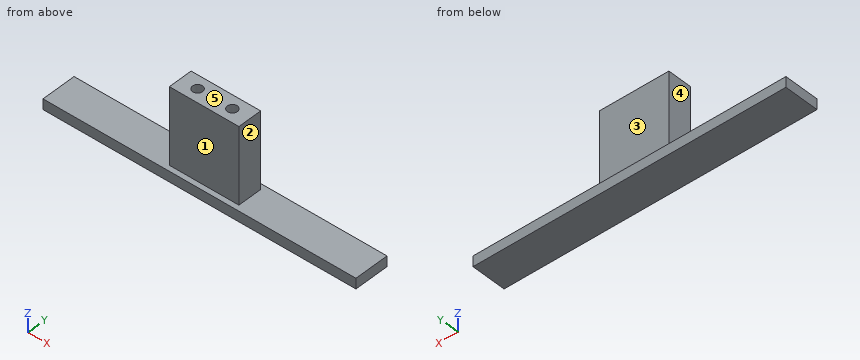
```python
from build123d import *

# Parameters (mm, degrees)
SKETCH_1_W          = 90
SKETCH_1_H          = 10
EXTRUDE_1_DEPTH     = 3
SKETCH_2_W          = 20
SKETCH_2_H          = 7
EXTRUDE_3_DEPTH     = 22
CUT_EXTRUDE_1_DEPTH = 9


with BuildPart() as part:
    # 草图1 → 凸台-拉伸1 (new body)
    with BuildSketch(Plane.XY):
        with Locations((45, 5)):
            Rectangle(SKETCH_1_W, SKETCH_1_H)
    extrude(amount=EXTRUDE_1_DEPTH)

    # 草图2 → 凸台-拉伸3 (add)
    with BuildSketch(Plane.XY.offset(3)):
        with Locations((45, 5)):
            Rectangle(SKETCH_2_W, SKETCH_2_H)
    extrude(amount=EXTRUDE_3_DEPTH)

    # 草图4 → 切除-拉伸1 (cut)
    with BuildSketch(Plane.XY.offset(25)):
        with BuildLine():
            ThreePointArc((48.55, 5), (50, 3.55), (51.45, 5))
            Line((51.45, 5), (50, 5))
            Line((50, 5), (48.55, 5))
        make_face()
        with BuildLine():
            Line((50, 5), (51.45, 5))
            ThreePointArc((51.45, 5), (50, 6.45), (48.55, 5))
            Line((48.55, 5), (50, 5))
        make_face()
        with BuildLine():
            ThreePointArc((48.55, 5), (50, 3.55), (51.45, 5))
            Line((51.45, 5), (50, 5))
            Line((50, 5), (48.55, 5))
        make_face()
        with BuildLine():
            Line((50, 5), (51.45, 5))
            ThreePointArc((51.45, 5), (50, 6.45), (48.55, 5))
            Line((48.55, 5), (50, 5))
        make_face()
        with BuildLine():
            ThreePointArc((38.55, 5), (40, 3.55), (41.45, 5))
            Line((41.45, 5), (40, 5))
            Line((40, 5), (38.55, 5))
        make_face()
        with BuildLine():
            Line((40, 5), (41.45, 5))
            ThreePointArc((41.45, 5), (40, 6.45), (38.55, 5))
            Line((38.55, 5), (40, 5))
        make_face()
        with BuildLine():
            ThreePointArc((38.55, 5), (40, 3.55), (41.45, 5))
            Line((41.45, 5), (40, 5))
            Line((40, 5), (38.55, 5))
        make_face()
        with BuildLine():
            Line((40, 5), (41.45, 5))
            ThreePointArc((41.45, 5), (40, 6.45), (38.55, 5))
            Line((38.55, 5), (40, 5))
        make_face()
    extrude(amount=-CUT_EXTRUDE_1_DEPTH, mode=Mode.SUBTRACT)


solid = part.part
```
CAD build for the part. Positions are in the model's coordinates, mm. Face numbers are marked on the shaded views. A direction names the side the tool comes from. Round coordinates to 2 decimals unless told otherwise and drop trailing zeros. Order: outer loops, then holes, each group sorted by start corner. A loop starts at its lowest first (then second) coordinate and runs counter-clockwise, first axis right, second up.
Item 1: Pin check, flat tips, straight feed: pin 1 (2 mm diameter, centred on y = 4.5, z = 11, fed in from -X); pin 2 (5 mm diameter, centred on x = 78.5, y = 7.5, fed in from +Z); pin 3 (0.9 mm diameter, centred on x = 40.5, y = 5, fed in from +Z). Stop position of each tip, or through.
Item 2: Saw through at A-A on x = 53. Write the cut outline in (y, z), then the cut area to 3 significant figures.
Item 3: Probe line 1 along X through (y, z) = (5, 23.25); line 2 along Y through (x, z) = (40, 19.5); line 3 along Z through (x, y) = (59, 4.25). List the from-to ranges inside material, lowest first.
Item 4: Saw through at C-C on z = 19.5. Write the cut outline in (x, y).
Item 5: Tool access for the marked faces 1, 2, 3, 4 and 5: list every direction of +Z, -Z, +X, -X, +Y, -Y with a clear straight run to the whole face (end or side of a thin tool).
Item 6: Saw through at D-D on z = 13.5. Write the cut outline in (x, y).
Item 7: Saw through at B-B on y = 5. Write the cut outline in (x, z), then the cut area to 3 significant figures.
Reported:
1. pin 1: stops at x = 35
1. pin 2: stops at z = 3
1. pin 3: stops at z = 16
2. outline: (0, 0) - (10, 0) - (10, 3) - (8.5, 3) - (8.5, 25) - (1.5, 25) - (1.5, 3) - (0, 3) - close
2. area: 184 mm2
3. line 1: x = 35 to 38.55, 41.45 to 48.55, 51.45 to 55
3. line 2: y = 1.5 to 3.55, 6.45 to 8.5
3. line 3: z = 0 to 3
4. outline: (35, 1.5) - (55, 1.5) - (55, 8.5) - (35, 8.5) - close; hole circle Ø2.9 at (40, 5); hole circle Ø2.9 at (50, 5)
5. face 1: +Z, +X, -X, -Y
5. face 2: +Z, +X, +Y, -Y
5. face 3: +Z, +X, -X, +Y
5. face 4: +Z, -X, +Y, -Y
5. face 5: +Z, +X, -X, +Y, -Y
6. outline: (35, 1.5) - (55, 1.5) - (55, 8.5) - (35, 8.5) - close
7. outline: (0, 0) - (90, 0) - (90, 3) - (55, 3) - (55, 25) - (51.45, 25) - (51.45, 16) - (48.55, 16) - (48.55, 25) - (41.45, 25) - (41.45, 16) - (38.55, 16) - (38.55, 25) - (35, 25) - (35, 3) - (0, 3) - close
7. area: 658 mm2
